Work out the finished part from the listing and answer in its coordinate system (mm). Face numbers are marked on the shaded views. A direction names the side the tool comes from. Give positions to 0.01 mm unless a question says otherwise; leave off trailing zeros. Loops run counter-clockwise (first coordinate to the right, second up) from the corner with the lowest first, then second, coordinate; pieces in that order, holes last. Notation, with made-up numbers: M -18,-7.75 L 6,-7.75 A26 cw 6,22.25 Z; hole C -0.75,-21 d11. An arc over 180 degrees is marked long. Answer as a JSON object with one key per item and string values. Group by question number.
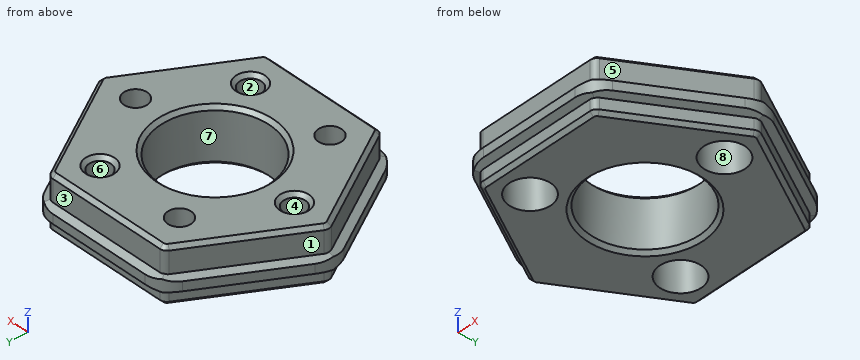
```python
from build123d import *

# Parameters (mm, degrees)
SKETCH_1_W                   = 32
SKETCH_1_H                   = 32
SKETCH_1_R                   = 7.5
EXTRUDE_1_DEPTH              = 3
SKETCH_23_W                  = 32
SKETCH_23_H                  = 32
SKETCH_23_R                  = 7.5
EXTRUDE_4_DEPTH              = 1.5
HOLE_WIZARD_M3_1_D           = 3.2
HOLE_WIZARD_M3_1_CBORE_D     = 5.7
HOLE_WIZARD_M3_1_CBORE_DEPTH = 5
F_3_0MM_1_D                  = 3
F_3_0MM_1_DEPTH              = 4
F_3_0MM_1_TIP                = 0.9012909285413404
SKETCH_26_OUTSIDE_W          = 43.174
SKETCH_26_OUTSIDE_H          = 43.174
SKETCH_26_OUTSIDE_R          = 15
CUT_EXTRUDE_1_DEPTH          = 24.837994882120434
EXTRUDE_5_DEPTH              = 7.5
FILLET_1_R                   = 1
CHAMFER_1_SIZE               = 0.5
FILLET_2_R                   = 4


with BuildPart() as part:
    # 草图1 → 凸台-拉伸1 (new, symmetric)
    with BuildSketch(Plane.XY):
        Rectangle(SKETCH_1_W, SKETCH_1_H)
        Circle(SKETCH_1_R, mode=Mode.SUBTRACT)
    extrude(amount=EXTRUDE_1_DEPTH, both=True)

    # 草图23 → 凸台-拉伸4 (add)
    with BuildSketch(Plane.XY.offset(3)):
        Rectangle(SKETCH_23_W, SKETCH_23_H)
        Circle(SKETCH_23_R, mode=Mode.SUBTRACT)
    extrude(amount=EXTRUDE_4_DEPTH)

    # M3 六角圆柱头螺钉的柱形沉头孔1 (through all)
    with Locations(Plane(origin=(0, 0, -3), x_dir=(-1, 0, 0), z_dir=(0, 0, -1))):
        with Locations((-12, 0), (6, 10.392304845), (6, -10.392304845)):
            CounterBoreHole(HOLE_WIZARD_M3_1_D / 2, HOLE_WIZARD_M3_1_CBORE_D / 2, HOLE_WIZARD_M3_1_CBORE_DEPTH)

    # Ø3.0mm 暗销孔1
    with Locations(Plane.XY.offset(4.500000000000001)):
        with Locations((-12, 0), (6, 10.392304845), (6, -10.392304845)):
            Hole(F_3_0MM_1_D / 2, depth=F_3_0MM_1_DEPTH)
            with Locations((0, 0, -(F_3_0MM_1_DEPTH + F_3_0MM_1_TIP / 2))):  # 118° drill point
                Cone(0, F_3_0MM_1_D / 2, F_3_0MM_1_TIP, mode=Mode.SUBTRACT)

    # 草图26 outside → 切除-拉伸1 (cut, through all)
    with BuildSketch(Plane(origin=(0, 0, -3), x_dir=(-1, 0, 0), z_dir=(0, 0, -1))):
        Rectangle(SKETCH_26_OUTSIDE_W, SKETCH_26_OUTSIDE_H)
        Circle(SKETCH_26_OUTSIDE_R, mode=Mode.SUBTRACT)
    extrude(amount=-CUT_EXTRUDE_1_DEPTH, mode=Mode.SUBTRACT)

    # 草图42 → 凸台-拉伸5 (add)
    with BuildSketch(Plane(origin=(0, 0, -3), x_dir=(-1, 0, 0), z_dir=(0, 0, -1))):
        with BuildLine():
            Line((-12.990381096299085, 7.499999931527694), (-17.32050807568877, 0))
            Line((-17.32050807568877, 0), (-12.99038117476846, -7.4999997956147455))
            ThreePointArc((-12.990381174768459, -7.499999795614747), (-15, 7.84693795e-08), (-12.990381096299085, 7.499999931527694))
        make_face()
        with BuildLine():
            ThreePointArc((-3.268098068e-08, -15), (-7.500000116343906, -12.990380989595394), (-12.990381174768459, -7.499999795614747))
            Line((-12.99038117476846, -7.4999997956147455), (-8.660254037844386, -15))
            Line((-8.660254037844386, -15), (-3.268098148e-08, -15))
        make_face()
        with BuildLine():
            Line((-8.660254037844389, 15), (-12.990381096299085, 7.499999931527694))
            ThreePointArc((-12.990381096299085, 7.499999931527694), (-7.500000044953584, 12.990381030812616), (-2.475085045e-08, 15))
            Line((-2.475085026e-08, 15), (-8.660254037844389, 15))
        make_face()
        with BuildLine():
            ThreePointArc((12.990381096299007, -7.499999931527828), (7.500000020084812, -12.990381045170608), (-3.268098068e-08, -15))
            Line((-3.268098148e-08, -15), (8.660254037844389, -15.000000000000002))
            Line((8.660254037844389, -15.000000000000002), (12.990381096299007, -7.499999931527833))
        make_face()
        with BuildLine():
            Line((8.660254037844386, 15.000000000000002), (-2.475085026e-08, 15))
            ThreePointArc((-2.475084712e-08, 15), (7.499999977454134, 12.990381069783442), (12.990381043108282, 7.500000023656865))
            Line((12.990381043108282, 7.500000023656862), (8.660254037844386, 15.000000000000002))
        make_face()
        with BuildLine():
            ThreePointArc((12.990381043108284, 7.500000023656865), (15, 5.319072383e-08), (12.990381096299007, -7.499999931527828))
            Line((12.990381096299007, -7.499999931527833), (17.320508075688775, -5.33e-15))
            Line((17.320508075688775, -5.2e-15), (12.990381043108282, 7.500000023656862))
        make_face()
    extrude(amount=-EXTRUDE_5_DEPTH)

    # 扫描1: sweep along a path in 草图44
    with BuildLine(Plane(origin=(0, 0, -1), x_dir=(-1, 0, 0), z_dir=(0, 0, -1))) as sweep_1_path:
        Line((-8.660254037844389, 15.000000000000002), (-17.32050807568877, -1.73e-15))
        Line((-17.32050807568877, -1.73e-15), (-8.660254037844387, -15))
        Line((-8.660254037844387, -15), (8.660254037844389, -15.000000000000004))
        Line((8.660254037844389, -15.000000000000004), (17.320508075688775, -6.07e-15))
        Line((17.320508075688775, -6.07e-15), (8.660254037844387, 15))
        Line((8.660254037844387, 15), (-8.660254037844389, 15.000000000000002))
    # 草图43 → 扫描1 (sweep)
    with BuildSketch(Plane(origin=(0, 0, 0), x_dir=(0, 0, -1), z_dir=(1, 0, 0))):
        Polygon((-0.9999999999999974, 15.000000000000002), (1, 15.000000000000002), (0.6360297657338008, 16), (-0.6360297657337987, 16), align=None)
    sweep(path=sweep_1_path.line, transition=Transition.RIGHT)

    # 圆角1
    fillet_1_edges = [part.edges().sort_by_distance(p)[0] for p in [
        (-8.660254037844386, 15.000000000000002, 2.7499999999999982),
        (-17.320508075688775, -5.27e-15, 2.7499999999999982),
        (-8.660254037844389, -15.000000000000002, 2.7499999999999982),
        (8.660254037844386, -15, 2.7499999999999982),
        (17.32050807568877, 0, 2.7499999999999982),
        (17.32050807568877, 0, -2),
        (8.660254037844386, -15, -2),
        (-8.660254037844389, -15.000000000000002, -2),
        (-17.320508075688775, -5.27e-15, -2),
        (-8.660254037844386, 15.000000000000002, -2),
        (8.660254037844389, 15, -2),
        (8.660254037844389, 15, 2.7499999999999982),
    ]]
    fillet(fillet_1_edges, radius=FILLET_1_R)

    # 倒角1
    chamfer_1_edges = [part.edges().sort_by_distance(p)[0] for p in [
        (-7.5, 4.25e-15, -3),
        (3.55e-15, 15, 4.5),
        (12.99038105676658, 7.5, 4.5),
        (12.990381056766578, -7.5, 4.5),
        (-12.99038105676658, 7.5, 4.5),
        (-12.990381056766584, -7.500000000000003, 4.5),
        (-1.78e-15, -15, 4.5),
        (-17.165807537309526, -4.64e-15, 4.5),
        (-8.582903768654763, -14.866025403784437, 4.5),
        (8.58290376865476, -14.86602540378444, 4.5),
        (-8.582903768654756, 14.866025403784443, 4.5),
        (17.16580753730952, 1.09e-15, 4.5),
        (-7.5, 4.25e-15, 4.5),
        (8.582903768654763, 14.866025403784437, 4.5),
        (3.55e-15, 15, -3),
        (12.99038105676658, 7.5, -3),
        (12.990381056766578, -7.5, -3),
        (-1.78e-15, -15, -3),
        (-12.990381056766584, -7.500000000000003, -3),
        (-12.99038105676658, 7.5, -3),
        (-17.165807537309526, -4.64e-15, -3),
        (-8.582903768654763, -14.86602540378444, -3),
        (8.58290376865476, -14.866025403784437, -3),
        (-8.582903768654756, 14.866025403784443, -3),
        (17.16580753730952, 1.11e-15, -3),
        (8.582903768654763, 14.866025403784437, -3),
        (7.5, -10.392304845, 4.5),
        (7.5, 10.392304845, 4.5),
        (-10.5, 1.8e-16, 4.5),
    ]]
    chamfer(chamfer_1_edges, length=CHAMFER_1_SIZE)

    # 圆角2
    fillet_2_edges = [part.edges().sort_by_distance(p)[0] for p in [
        (9.237604307034012, -16, -1.11e-15),
        (18.475208614068023, -4.33e-15, -1.11e-15),
        (-9.23760430703402, -16, -1.11e-15),
        (9.23760430703402, 16, -1.11e-15),
        (-18.475208614068023, 3.03e-15, -1.11e-15),
        (-9.23760430703401, 16, -1.11e-15),
    ]]
    fillet(fillet_2_edges, radius=FILLET_2_R)


solid = part.part
```
Item 1: A cutting plane is placed at D-D (y = -1). Give the number of separate pieces and of enclosed holes in the cut face, and give its area (3 significant figures).
Item 2: Find the intervals of material crossed by probe 1 along Y at (x, z) = (-6, -1.8); probe 2 along Y at (x, z) = (6, 1.85); probe 3 along X at (y, z) = (-0.5, 3), in increasing order. Write a range as [from, to].
Item 3: A cutting plane is placed at A-A (x = 0). Determine the outline of the cut face in (y, z), and give its area (3 significant figures).
Item 4: A tool of negligible diameter and unlimited length cuts with its end or side. For the marked faces 5, 6, 7 and 8, from which of +Z, -Z, +X, -X, +Y, -Y can it reach the whole face along a straight path? Write none if from no direction.
Item 5: For a pull along X with two mould halves and no side action, classify the marked faces 1, 2, 3 and 4 as pulls with the +X half, pulls with the -X half, needs draft (parallel to the pull), parting line crosses it, or undercut.
Item 6: A cutting plane is placed at B-B (z = -1.75). Determine the outline of the cut face in (x, y).
Item 7: Given pin 1 Ø5 at (x, y) = (-13.5, -11) entering from +Z; pin 2 Ø0.8 at (x, z) = (1, -2) entering from +Y; pin 3 Ø1.9 at (x, y) = (-6, 10.39) entering from +Z; pin 4 Ø3 at (x, y) = (-5.5, 11.5) entering from -Z, each flat-ended and moving along its own axis, determine where each tip first touches the part or whether it passes through.
Item 8: A cutting plane is placed at C-C (x = 10). Determine the outline of the cut face in (y, z), and give its area (3 significant figures).
The answers:
{
 "1": {"separate pieces": "3", "enclosed holes": "0", "area": "99.3 mm^2"},
 "2": {"probe 1": "y = [-15, -13.24], [-7.54, -4.5], [4.5, 7.54], [13.24, 15]", "probe 2": "y = [-15, -11.89], [-8.89, -4.5], [4.5, 8.89], [11.89, 15]", "probe 3": "x = [-17.03, -13.41], [-10.59, -7.48], [7.48, 10.48], [13.52, 17.03]"},
 "3": {"outline": "M -16,-0.64 L -15,-1 L -15,-2.5 L -14.5,-3 L -8,-3 L -7.5,-2.5 L -7.5,4 L -8,4.5 L -14.5,4.5 L -15,4 L -15,1 L -16,0.64 Z; M 7.5,-2.5 L 8,-3 L 14.5,-3 L 15,-2.5 L 15,-1 L 16,-0.64 L 16,0.64 L 15,1 L 15,4 L 14.5,4.5 L 8,4.5 L 7.5,4 Z", "area": "115 mm^2"},
 "4": {"face 5": "+Z, +X, -Y", "face 6": "+Z", "face 7": "+Z, -Z", "face 8": "-Z"},
 "5": {"face 1": "pulls with the -X half", "face 2": "undercut", "face 3": "needs draft", "face 4": "undercut"},
 "6": {"outline": "M -17.03,-0.5 L -8.95,-14.5 A1 ccw -8.08,-15 L 8.08,-15 A1 ccw 8.95,-14.5 L 17.03,-0.5 A1 ccw 17.03,0.5 L 8.95,14.5 A1 ccw 8.08,15 L -8.08,15 A1 ccw -8.95,14.5 L -17.03,0.5 A1 ccw Z; hole C -6,-10.39 d5.7; hole C -6,10.39 d5.7; hole C 0,0 d15; hole C 12,0 d5.7"},
 "7": {"pin 1": "stops at z = 4.31", "pin 2": "stops at y = 15", "pin 3": "passes through", "pin 4": "stops at z = 2"},
 "8": {"outline": "M -14.56,-0.66 L -12.68,-1 L -12.68,-2.5 L -11.68,-3 L -2.03,-3 L -2.03,2 L 2.03,2 L 2.03,-3 L 11.68,-3 L 12.68,-2.5 L 12.68,-1 L 14.56,-0.66 L 14.56,0.66 L 12.68,1 L 12.68,4 L 11.68,4.5 L -11.68,4.5 L -12.68,4 L -12.68,1 L -14.56,0.66 Z", "area": "175 mm^2"}
}
